Geometry check sheet. Reference: the model listing, model coordinates, mm. Face numbers are marked on the shaded views. Give positions to 0.01 mm unless a question says otherwise; leave off trailing zeros. Write each loop counter-clockwise with the first axis right and the second up, starting at its lowest first coordinate (ties: lowest second). Pieces come first, ordered by that corner, then holes. Notation, with made-up numbers: (5.5, 19.5) -> (63.5, 19.5) arc R27 ccw to (63.5, 55.5) -> close; hole circle Ø2 at (-27.75, 67). An arc over 180 degrees is marked (long way). Use a Markdown table: item, result. Add a question column.
from build123d import *

# Parameters (mm, degrees)
SKETCH1_W                   = 18
SKETCH1_H                   = 60
SKETCH1_R                   = 3
BOSS_EXTRUDE1_DEPTH         = 38
CHAMFER1_SIZE               = 2
CUT_EXTRUDE1_DEPTH          = 38
M12X1_25_TAPPED_HOLE1_D     = 12
M12X1_25_TAPPED_HOLE1_DEPTH = 20
M12X1_25_TAPPED_HOLE1_TIP   = 3.464101615


with BuildPart() as part:
    # Sketch1 → Boss-Extrude1 (new body)
    with BuildSketch(Plane(origin=(0, 0, 0), x_dir=(0, 0, -1), z_dir=(1, 0, 0))):
        Rectangle(SKETCH1_W, SKETCH1_H)
        with Locations((0, 23)):
            Circle(SKETCH1_R, mode=Mode.SUBTRACT)
    extrude(amount=-BOSS_EXTRUDE1_DEPTH)

    # Chamfer1
    chamfer1_edges = [part.edges().sort_by_distance(p)[0] for p in [
        (-38, 30, 0),
        (0, 30, 0),
        (-19, 30, 9),
        (-19, 30, -9),
    ]]
    chamfer(chamfer1_edges, length=CHAMFER1_SIZE)

    # Sketch2 → Cut-Extrude1 (cut)
    with BuildSketch(Plane.XY.offset(9)):
        Polygon((-32.75, -30), (-32.75, -27.5), (-30.25, -27.5), (-30.25, -25), (-27.75, -25), (-27.75, -22.5), (-25.25, -22.5), (-25.25, -20), (-22.75, -20), (-22.75, -17.5), (-20.25, -17.5), (-20.25, -15), (-17.75, -15), (-17.75, -17.5), (-15.25, -17.5), (-15.25, -20), (-12.75, -20), (-12.75, -22.5), (-10.25, -22.5), (-10.25, -25), (-7.75, -25), (-7.75, -27.5), (-5.25, -27.5), (-5.25, -30), align=None)
    extrude(amount=-CUT_EXTRUDE1_DEPTH, mode=Mode.SUBTRACT)

    # M12x1.25 Tapped Hole1
    with Locations(Plane(origin=(0, 30, 0), x_dir=(1, 0, 0), z_dir=(0, 1, 0))):
        with Locations((-19, 0)):
            Hole(M12X1_25_TAPPED_HOLE1_D / 2, depth=M12X1_25_TAPPED_HOLE1_DEPTH)
            with Locations((0, 0, -(M12X1_25_TAPPED_HOLE1_DEPTH + M12X1_25_TAPPED_HOLE1_TIP / 2))):  # 120° drill point
                Cone(0, M12X1_25_TAPPED_HOLE1_D / 2, M12X1_25_TAPPED_HOLE1_TIP, mode=Mode.SUBTRACT)


solid = part.part
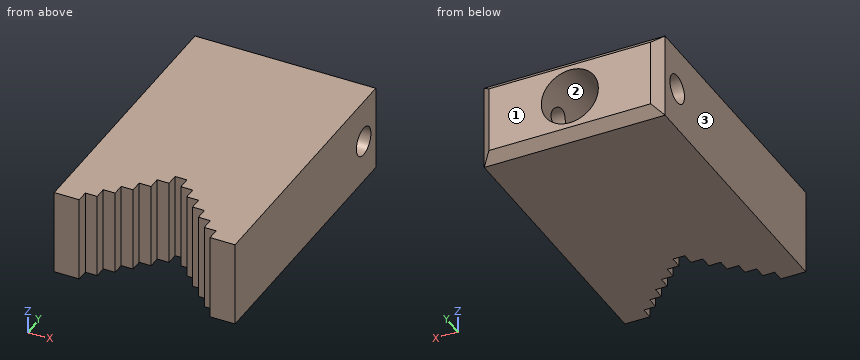
1) Sectioned sample at A-A, the plane y = -16.5. Enter the section's corners in (x, z).
2) Material ranges on probe 1 along Z at (x, y) = (-35, 23); probe 2 along Y at (x, z) = (-33, 0); probe 3 along Y at (x, z) = (-29.75, 0), recorded low to high. Write a range as [from, to].
3) Draft check along X on the marked faces 1, 2 and 3. Enter one of: +X half, -X half, draft (parallel to the pull), parting line (faces both ways), or undercut.
4) Gauge pin test, flat ends, axial feed: P1, Ø1, axis at x = -22, z = -4.5, coming from the +Y side; P2, Ø3, axis at x = -19, z = 0.5, coming from the -Y side; P3, Ø2, axis at x = -6.5, z = 4.5, coming from the -Y side. Record the tip position at first contact, or that the pin passes through.
5) Sectioned sample at B-B, the plane y = 16. Enter the section's corners in (x, z).
6) Sectioned sample at D-D, the plane y = 23. Enter the section's corners in (x, z).
7) Sectioned sample at C-C, the plane x = -7. Enter the section's corners in (y, z).
Check values:
| question | item | result |
|---|---|---|
| 1 | outline | (-38, -9) -> (-20.25, -9) -> (-20.25, 9) -> (-38, 9) -> close; (-17.75, -9) -> (0, -9) -> (0, 9) -> (-17.75, 9) -> close |
| 2 | probe 1 | [-9, -3], [3, 9] |
| 2 | probe 2 | [-30, 20], [26, 30] |
| 2 | probe 3 | [-25, 20], [26, 30] |
| 3 | face 1 | draft |
| 3 | face 2 | undercut |
| 3 | face 3 | -X half |
| 4 | P1 | y = 9.95 |
| 4 | P2 | y = -17.5 |
| 4 | P3 | y = -27.5 |
| 5 | outline | (-38, -9) -> (0, -9) -> (0, 9) -> (-38, 9) -> close; hole circle Ø12 at (-19, 0) |
| 6 | outline | (-38, -9) -> (0, -9) -> (0, -3) -> (-13.8, -3) arc R6 cw to (-24.2, -3) -> (-38, -3) -> close; (-38, 3) -> (-24.2, 3) arc R6 cw to (-13.8, 3) -> (0, 3) -> (0, 9) -> (-38, 9) -> close |
| 7 | outline | (-27.5, -9) -> (28, -9) -> (30, -7) -> (30, 7) -> (28, 9) -> (-27.5, 9) -> close; hole circle Ø6 at (23, 0) |
